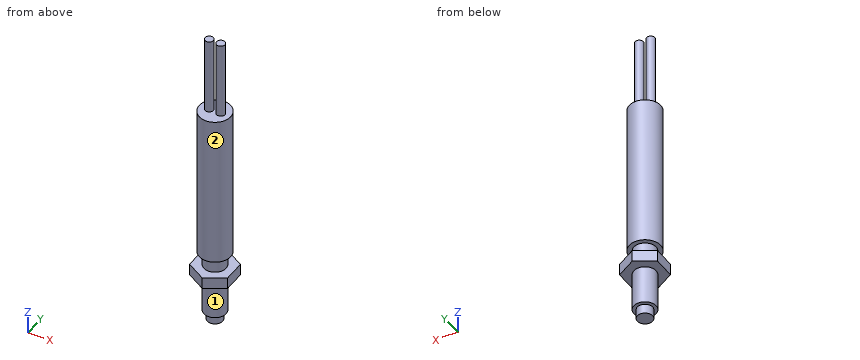
from build123d import *

# Parameters (mm, degrees)
ESQUISSE1_R        = 2.9
BOSS_EXTRU_1_DEPTH = 16.8
ESQUISSE2_R        = 2
BOSS_EXTRU_2_DEPTH = 2.5
ESQUISSE3_R        = 4.1
BOSS_EXTRU_3_DEPTH = 40
ESQUISSE4_R        = 1.1
BOSS_EXTRU_4_DEPTH = 20
BOSS_EXTRU_5_START = 10
BOSS_EXTRU_5_DEPTH = 3


with BuildPart() as part:
    # Esquisse1 → Boss.-Extru.1 (new body)
    with BuildSketch(Plane.XY):
        Circle(ESQUISSE1_R)
    extrude(amount=BOSS_EXTRU_1_DEPTH)

    # Esquisse2 → Boss.-Extru.2 (add)
    with BuildSketch(Plane(origin=(0, 0, 0), x_dir=(-1, 0, 0), z_dir=(0, 0, -1))):
        Circle(ESQUISSE2_R)
    extrude(amount=BOSS_EXTRU_2_DEPTH)

    # Esquisse3 → Boss.-Extru.3 (add)
    with BuildSketch(Plane.XY.offset(16.8)):
        Circle(ESQUISSE3_R)
    extrude(amount=BOSS_EXTRU_3_DEPTH)

    # Esquisse4 → Boss.-Extru.4 (add)
    with BuildSketch(Plane.XY.offset(56.8)):
        with Locations((-1.5, 0)):
            Circle(ESQUISSE4_R)
        with Locations(Location((1.5, 0, 0), (0, 0, 180))):
            Circle(ESQUISSE4_R)
    extrude(amount=BOSS_EXTRU_4_DEPTH)

    # Esquisse5 → Boss.-Extru.5 (add)
    with BuildSketch(Plane.XY.offset(BOSS_EXTRU_5_START)):
        Polygon((0, -5.715767665), (4.95, -2.857883832), (4.95, 2.857883832), (0, 5.715767665), (-4.95, 2.857883832), (-4.95, -2.857883832), align=None)
    extrude(amount=BOSS_EXTRU_5_DEPTH)


solid = part.part
The model under review builds one solid part; all positions refer to its coordinate system, in mm. Face numbers are marked on the shaded views. A direction names the side the tool comes from. Round coordinates to 2 decimals unless told otherwise and drop trailing zeros. Write each loop counter-clockwise with the first axis right and the second up, starting at its lowest first coordinate (ties: lowest second). Pieces come first, ordered by that corner, then holes. Notation, with made-up numbers: (-2.75, 28.5) -> (3.25, 28.5) arc R23 cw to (3.25, 63.5) -> close; hole circle Ø1 at (53, -14). An arc over 180 degrees is marked (long way). Answer as a JSON object with one key per item and string values.
1. We need section B-B on z = 42. State the section outline as (x, y) points, and give its area (3 significant figures).
Results found:
{"outline": "circle Ø8.2 at (0, 0)", "area": "52.8 mm^2"}
2. We need section A-A on y = 0. State the section outline as (x, z) points.
Results found:
{"outline": "(-4.95, 10) -> (-2.9, 10) -> (-2.9, 0) -> (-2, 0) -> (-2, -2.5) -> (2, -2.5) -> (2, 0) -> (2.9, 0) -> (2.9, 10) -> (4.95, 10) -> (4.95, 13) -> (2.9, 13) -> (2.9, 16.8) -> (4.1, 16.8) -> (4.1, 56.8) -> (2.6, 56.8) -> (2.6, 76.8) -> (0.4, 76.8) -> (0.4, 56.8) -> (-0.4, 56.8) -> (-0.4, 76.8) -> (-2.6, 76.8) -> (-2.6, 56.8) -> (-4.1, 56.8) -> (-4.1, 16.8) -> (-2.9, 16.8) -> (-2.9, 13) -> (-4.95, 13) -> close"}
3. Clearance check with flat-ended pins moving along their axes: pin 1 (2 mm diameter, centred on x = -0.5, z = 61, fed in from +Y); pin 2 (1 mm diameter, centred on x = 0.5, z = 52.5, fed in from +Y); pin 3 (3 mm diameter, centred on y = -2, z = 60, fed in from +X). State where each tip first meets the part, or that it passes through.
Results found:
{"pin 1": "stops at y = 1.1", "pin 2": "stops at y = 4.1", "pin 3": "stops at x = 2.48"}
4. Machinability: for the marked faces 1 and 2, which of the approach directions +Z, -Z, +X, -X, +Y, -Y give a long, thin tool a straight path to every point of the face, cutting with its end or side? Answer none if there is none.
Results found:
{"face 1": "-Z", "face 2": "+Z"}
5. To check wall thickness, follow line 1 along Z through (x, y) = (2.5, 2.75); line 2 along X through (y, z) = (0.5, 6); line 3 along Z through (x, y) = (-0.25, 1.5). State the ranges of each line that lie inside material, in increasing order.
Results found:
{"line 1": "z = 10 to 13, 16.8 to 56.8", "line 2": "x = -2.86 to 2.86", "line 3": "z = -2.5 to 56.8"}
6. We need section C-C on y = 5. State the section outline as (x, z) points.
Results found:
{"outline": "(-1.24, 10) -> (1.24, 10) -> (1.24, 13) -> (-1.24, 13) -> close"}
